Here's how the part is built. I have some questions about the finished solid (model axes, mm). Face numbers are marked on the shaded views. A direction names the side the tool comes from. Round coordinates to 2 decimals unless told otherwise and drop trailing zeros. Write each loop counter-clockwise with the first axis right and the second up, starting at its lowest first coordinate (ties: lowest second). Pieces come first, ordered by that corner, then holes. Notation, with made-up numbers: M 5.5,49.25 L 58.5,49.25 A22 cw 58.5,77.25 Z; hole C 58,38 d2. An arc over 180 degrees is marked long. Use one line per item in the form item = value. Start each with the question number.
Q1. I need wall thicknesses on line 1 along Z through (x, y) = (0, 1.8); line 2 along Z through (x, y) = (-1.75, -1.5); line 3 along X through (y, z) = (-1.65, -0.25). Which ranges of each line are inside material? Lowest first, please. Write a range as from..to.
Q2. We'd pull the mould along Z, two halves only. Please class the marked faces 3, 4, 5 and 6: +Z half, -Z half, draft (parallel to the pull), parting line (faces both ways), or undercut.
Q3. I want a section at A-A on z = 0. List the corners of the cut face in (x, y) for me.
Q4. I want a section at B-B on x = 0. List the corners of the cut face in (y, z) for me.
Q5. For the marked faces 1 and 2, which set-ups out of +Z, -Z, +X, -X, +Y, -Y let a thin tool reach every point of the face, with its end or its side?
Q6. I'm going to push flat-ended pins straight in: pin 1 Ø2 at (y, z) = (1, -3) entering from +X; pin 2 Ø1.5 at (x, y) = (-3, -0.5) entering from +Z; pin 3 Ø1 at (x, y) = (2, -1.5) entering from +Z; pin 4 Ø4 at (x, z) = (0, 0) entering from +Y. Where does each tip first touch, or does it pass through?
Q7. I want a section at D-D on y = -0.8. List the corners of the cut face in (x, z) for me.
Q8. I want a section at C-C on y = 1.45. List the corners of the cut face in (x, z) for me, and give its area (3 significant figures).
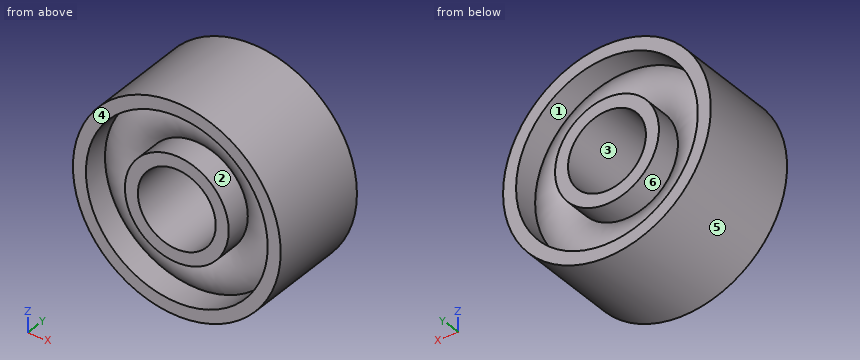
```python
from build123d import *


with BuildPart() as part:
    # Sketch1 → Revolve1 (revolve)
    with BuildSketch(Plane.XY):
        with BuildLine():
            Line((1.5, 2), (1.5, -2))
            Line((1.5, -2), (2, -2))
            Line((2, -2), (2, -1))
            ThreePointArc((2, -1), (2.75, -1.25), (3.5, -1))
            Line((3.5, -1), (3.5, -2))
            Line((3.5, -2), (4, -2))
            Line((4, -2), (4, 2))
            Line((4, 2), (3.5, 2))
            Line((3.5, 2), (3.5, 1))
            ThreePointArc((3.5, 1), (2.75, 1.25), (2, 1))
            Line((2, 1), (2, 2))
            Line((2, 2), (1.5, 2))
        make_face()
    revolve(axis=Axis((0, 1.338212484, 0), (0, -1, 0)))


solid = part.part
```
Reported:
q1.line_1 = -4..-3.5, -2..-1.5, 1.5..2, 3.5..4
q1.line_2 = -3.6..-3.03, -0.97..0.97, 3.03..3.6
q1.line_3 = -3.99..-3.49, -1.98..-1.48, 1.48..1.98, 3.49..3.99
q2.face_3 = undercut
q2.face_4 = draft
q2.face_5 = parting line
q2.face_6 = undercut
q3.outline = M -4,-2 L -3.5,-2 L -3.5,-1 A1.25 ccw -2,-1 L -2,-2 L -1.5,-2 L -1.5,2 L -2,2 L -2,1 A1.25 ccw -3.5,1 L -3.5,2 L -4,2 Z; M 1.5,-2 L 2,-2 L 2,-1 A1.25 ccw 3.5,-1 L 3.5,-2 L 4,-2 L 4,2 L 3.5,2 L 3.5,1 A1.25 ccw 2,1 L 2,2 L 1.5,2 Z
q4.outline = M -2,-4 L 2,-4 L 2,-3.5 L 1,-3.5 A1.25 ccw 1,-2 L 2,-2 L 2,-1.5 L -2,-1.5 L -2,-2 L -1,-2 A1.25 ccw -1,-3.5 L -2,-3.5 Z; M -2,1.5 L 2,1.5 L 2,2 L 1,2 A1.25 ccw 1,3.5 L 2,3.5 L 2,4 L -2,4 L -2,3.5 L -1,3.5 A1.25 ccw -1,2 L -2,2 Z
q5.face_1 = +Y
q5.face_2 = -Y
q6.pin_1 = 3.46
q6.pin_2 = 3.31
q6.pin_3 = 3.71
q6.pin_4 = 2
q7.outline = C 0,0 d8; hole C 0,0 d3
q8.outline = C 0,0 d8; C 0,0 d4; hole C 0,0 d7; hole C 0,0 d3
q8.area = 17.3 mm^2
